Geometry check sheet. Reference: drawing and pictorial views, mm from the part's lowest x, y, z. Round coordinates to 2 decimals unless told otherwise and drop trailing zeros. Write each loop counter-clockwise with the first axis right and the second up, starting at its lowest first coordinate (ties: lowest second). Pieces come first, ordered by that corner, then holes.
Item 1: Material ranges on line 1 along Z through (x, y) = (361.95, 1.1); line 2 along Y through (x, z) = (459, 19) (1 decimal), recorded low to high.
Item 2: Section check A-A, the plane x = 326. Record the cut outline in (y, z) (1 decimal), plus the area to 3 significant figures.
Item 3: Depth check by flat-ended pin: pin 1 (11 mm diameter, centred on x = 143.5, z = 14.5, fed in from +Y) (1 decimal); pin 2 (4 mm diameter, centred on x = 423.5, z = 4.5, fed in from +Y); pin 3 (3 mm diameter, centred on x = 266, y = 19.5, fed in from +Z) (1 decimal); pin 4 (4 mm diameter, centred on x = 120.65, z = 14.29, fed in from -Y). Enter the tip coordinate at first touch or a pass-through.
Item 4: Section check B-B, the plane y = 19.75. Record the cut outline in (x, z) (1 decimal).
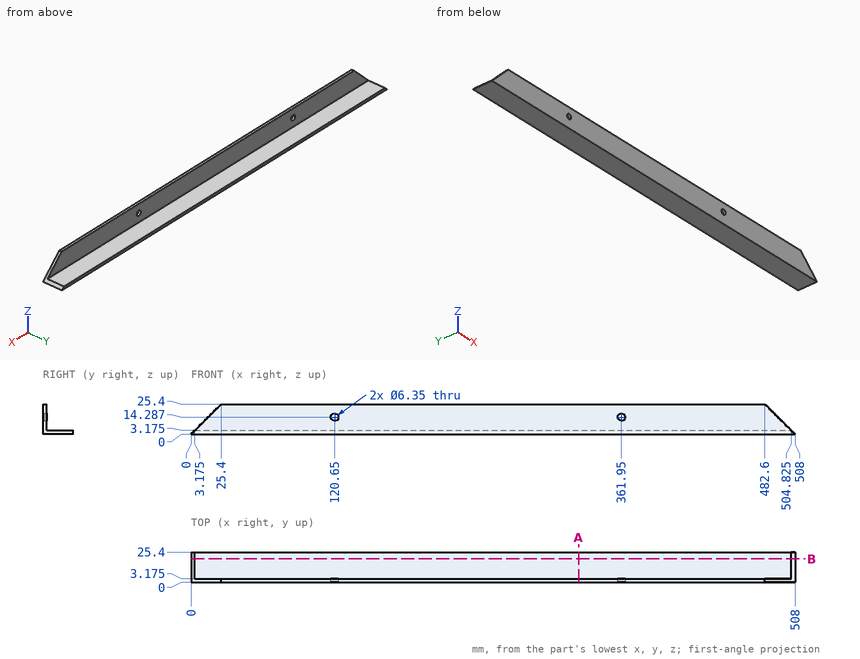
Values found:
1. line 1: z = 0 to 11.11, 17.46 to 25.4
1. line 2: y = 0 to 3.2
2. outline: (0, 0) - (25.4, 0) - (25.4, 3.2) - (3.2, 3.2) - (3.2, 25.4) - (0, 25.4) - close
2. area: 151 mm2
3. pin 1: stops at y = 3.2
3. pin 2: stops at y = 25.4
3. pin 3: stops at z = 3.2
3. pin 4: passes through
4. outline: (0, 0) - (508, 0) - (504.8, 3.2) - (3.2, 3.2) - close
